```python
from build123d import *

# Parameters (mm, degrees)
F0_R     = 2.25
F1_DEPTH = 8.3058
F2_R     = 2.032
F3_R     = 1.55
F4_DEPTH = 6.1214


with BuildPart() as f1:
    # F0 (on Top) → F1 (new body)
    with BuildSketch(Plane.XY):
        Circle(F0_R)
    extrude(amount=F1_DEPTH)

    # F2
    f2_edges = [f1.edges().sort_by_distance(p)[0] for p in [
        (-2.25, 0, 8.3058),
    ]]
    fillet(f2_edges, radius=F2_R)

    # F3 (on face) → F4 (cut)
    with BuildSketch(Plane(origin=(0, 0, 0), x_dir=(1, 0, 0), z_dir=(0, 0, -1))):
        Circle(F3_R)
    extrude(amount=-F4_DEPTH, mode=Mode.SUBTRACT)


solid = f1.part
```
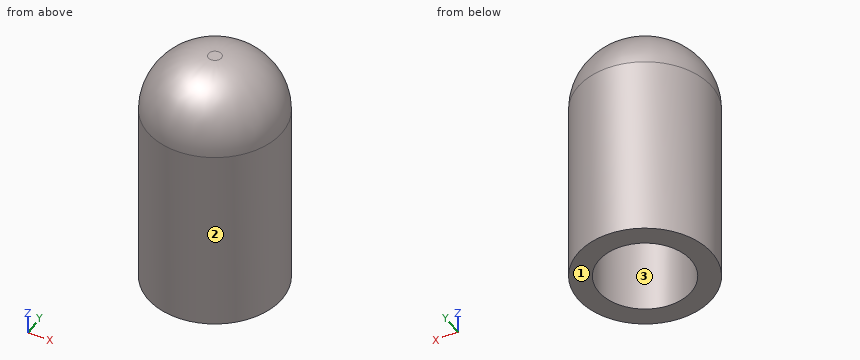
Here's how the part is built. I have some questions about the finished solid (model axes, mm). Face numbers are marked on the shaded views. Coordinates: 2 decimals unless noted, no trailing zeros. Loops run counter-clockwise (first coordinate to the right, second up) from the corner with the lowest first, then second, coordinate; pieces in that order, holes last. Notation, with made-up numbers: (-25, 7) -> (24, 7) arc R15 ccw to (24, 36) -> close; hole circle Ø10 at (17.25, 69.5). An arc over 180 degrees is marked (long way). Return JSON: item names as keys, results as strings.
1) Will these pins go through, and if not, where does the flat tip stop? pin 1 (2 mm diameter, centred on y = 1.5, z = 7, fed in from +X); pin 2 (1.6 mm diameter, centred on x = 0.5, y = -0.5, fed in from -Z); pin 3 (1.5 mm diameter, centred on x = 0.5, z = 3, fed in from -Y).
Results below:
{"pin 1": "x = 2.15", "pin 2": "z = 6.12", "pin 3": "y = -2.25"}
2) If we section it at A-A, the plane z = 4.75: Write out the boundary of the cut face in (x, y).
Results below:
{"outline": "circle Ø4.5 at (0, 0); hole circle Ø3.1 at (0, 0)"}
3) Thinking about a two-plate mould opening in Y: for the marked faces 1, 2 and 3, which applies, +Y half, -Y half, draft (parallel to the pull), parting line (faces both ways), or undercut?
Results below:
{"face 1": "draft", "face 2": "parting line", "face 3": "undercut"}
4) I need wall thicknesses on line 1 (Y direction, x = 0, z = 3.5); line 2 (X direction, y = 0.7, z = 5.5); line 3 (Y direction, x = -0.8, z = 5.25). Which ranges of each line are inside material? Lowest first, please. Write a range as from..to.
Results below:
{"line 1": "-2.25..-1.55, 1.55..2.25", "line 2": "-2.14..-1.38, 1.38..2.14", "line 3": "-2.1..-1.33, 1.33..2.1"}
